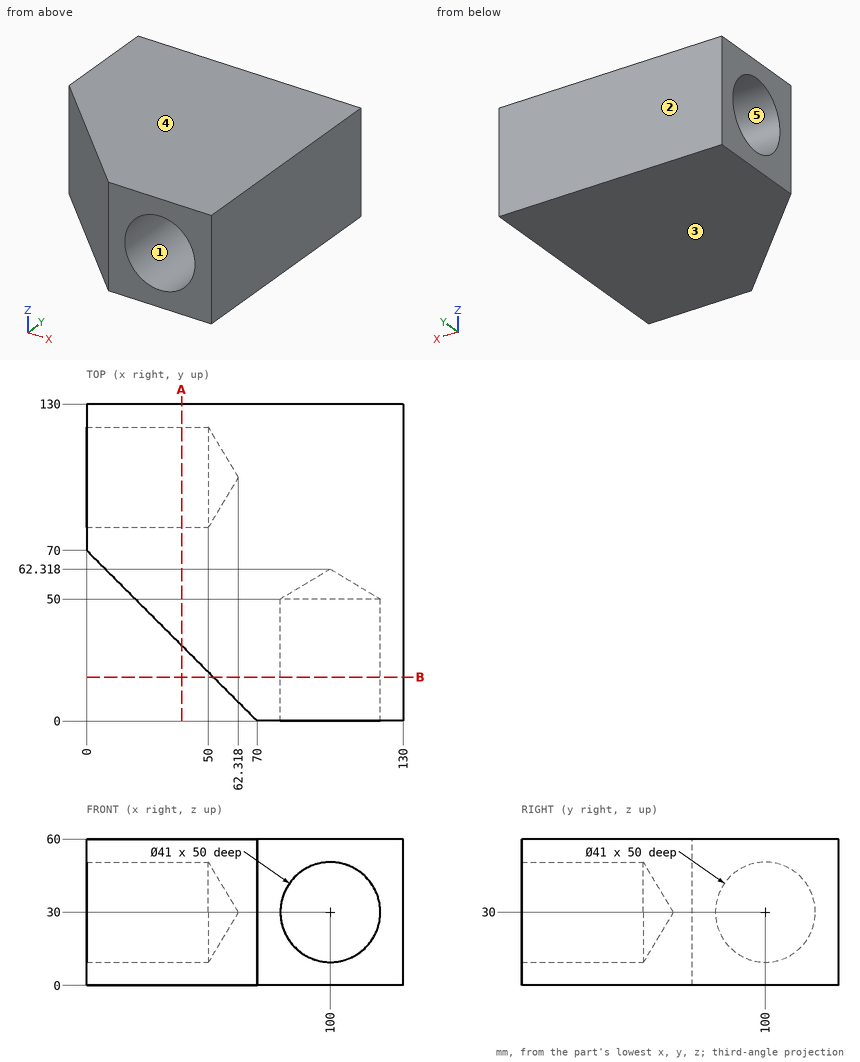
Answer from the drawing. Dimensions are ordinates in mm from the lowest x, y and z of the part. A direction names the side the tool comes from. Coordinates: 2 decimals unless noted, no trailing zeros. Write each loop counter-clockwise with the first axis right and the second up, starting at its lowest first coordinate (ties: lowest second). Pieces come first, ordered by that corner, then holes. Notation, with made-up numbers: (26, 84.25) - (54, 84.25) arc R12 cw to (54, 97.25) - close; hole circle Ø5 at (11, 64.5). An arc over 180 degrees is marked (long way). Return JSON: item names as keys, results as strings.
1. The part is cut by section B-B on y = 18. Determine the outline of the cut face in (x, z), then the cut area to 3 significant figures.
Final values:
{"outline": "(52, 0) - (130, 0) - (130, 60) - (52, 60) - close; hole circle Ø41 at (100, 30)", "area": "3,360 mm^2"}
2. For a pull along Z with two mould halves and no side action, classify the marked faces 1, 2 and 3 as +Z half, -Z half, draft (parallel to the pull), parting line (faces both ways), or undercut.
Final values:
{"face 1": "undercut", "face 2": "draft", "face 3": "-Z half"}
3. Consider line 1 along Z through (x, y) = (100, 18); line 2 along X through (y, z) = (37, 32.5) (1 decimal); line 3 along X through (y, z) = (48, 31) (1 decimal). Determine where each line is inside the solid, lowest interval first.
Final values:
{"line 1": "0 to 9.5, 50.5 to 60", "line 2": "33 to 79.7, 120.3 to 130", "line 3": "22 to 79.5, 120.5 to 130"}
4. Each of these flat-tipped pins is pushed along its axis until it touches: pin 1 Ø8 at (x, z) = (62.5, 53) entering from -Y; pin 2 Ø4 at (x, z) = (14.5, 51) entering from -Y; pin 3 Ø4 at (x, z) = (23, 53.5) entering from -Y. Where does it stop, or does it pass through?
Final values:
{"pin 1": "y = 3.5", "pin 2": "y = 53.5", "pin 3": "y = 45"}
5. Which of the six approach directions +Z, -Z, +X, -X, +Y, -Y give full straight-line access (tool end or side, diameter ignored) to the marked faces 4 and 5?
Final values:
{"face 4": "+Z, +X, -X, +Y, -Y", "face 5": "-X"}
6. The part is cut by section A-A on x = 39. Determine the outline of the cut face in (y, z), then the cut area to 3 significant figures.
Final values:
{"outline": "(31, 0) - (130, 0) - (130, 60) - (31, 60) - close; hole circle Ø41 at (100, 30)", "area": "4,620 mm^2"}
